Verification items for the finished model (mm, model axes). Face numbers are marked on the shaded views. A direction names the side the tool comes from. Give positions to 0.01 mm unless a question says otherwise; leave off trailing zeros. Order: outer loops, then holes, each group sorted by start corner. A loop starts at its lowest first (then second) coordinate and runs counter-clockwise, first axis right, second up. Notation, with made-up numbers: (25.5, 15.5) -> (66.5, 15.5) arc R19 ccw to (66.5, 41.5) -> close; hole circle Ø4 at (33, -15). An arc over 180 degrees is marked (long way). Return JSON: item names as keys, results as strings. Group by question number.
(1) Cross-section at D-D on z = 52. Enter the section's corners in (x, y).
(2) Cross-section at B-B on x = -13.5. Enter the section's corners in (y, z), then the cut area to 3 significant figures.
(3) Thickness scan on line 1 along Z through (x, y) = (-22.75, 37); line 2 along Y through (x, z) = (-16.75, 18); line 3 along Y through (x, z) = (-19.75, 10). Record the ranges inside material, lowest first.
(4) Cross-section at A-A on y = 11. Enter the section's corners in (x, z), then the cut area to 3 significant figures.
(5) Depth check by flat-ended pin: pin 1 Ø2 at (x, z) = (-17.5, 43.5) entering from +Y; pin 2 Ø9 at (x, y) = (-16.19, 27.83) entering from -Z; pin 3 Ø5 at (x, z) = (-17, 16.5) entering from +Y; pin 4 Ø12 at (x, z) = (-25, 61.5) entering from +Y. Enter the tip coordinate at first touch or a pass-through.
(6) Cross-section at C-C on z = 5. Enter the section's corners in (x, y), then the cut area to 3 significant figures.
(7) Tool access check on the marked faces 1 and 2. Record the directions out of +Z, -Z, +X, -X, +Y, -Y that give a thin tool (end or side, any length) a straight path to the whole face; none if there is none.
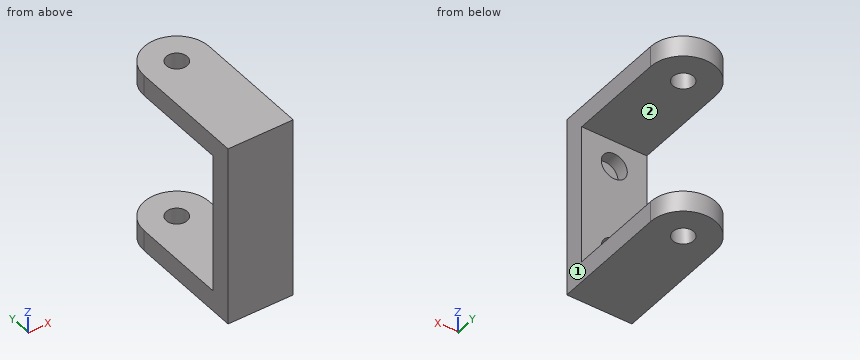
from build123d import *

# Parameters (mm, degrees)
IZIM1_W                     = 25
IZIM1_H                     = 57.5
Y_KSEKLIK_EKSTR_ZYON1_DEPTH = 70
RADYUS1_RADIUS              = 12.5
RADYUS1_LENGTH              = 70
IZIM3_W                     = 54
IZIM3_H                     = 49.5
KES_EKSTR_ZYON1_DEPTH       = 85.564510613
IZIM4_R                     = 5
KES_EKSTR_ZYON2_DEPTH       = 5
IZIM5_R                     = 4
KES_EKSTR_ZYON3_DEPTH       = 86.728971246


with BuildPart() as part:
    # Çizim1 → Yükseklik-Ekstrüzyon1 (new body)
    with BuildSketch(Plane.XY):
        with Locations((-16.193205739, 11.575630252)):
            Rectangle(IZIM1_W, IZIM1_H)
    extrude(amount=Y_KSEKLIK_EKSTR_ZYON1_DEPTH)

    # Radyus1: full round fillet: the end face becomes a half cylinder, R = half its width
    radyus1_face = Plane((-16.193205739, 40.325630252, 35), x_dir=(0, 0, 1), z_dir=(0, 1, 0))  # on the end face: x along it, z out of the body
    radyus1_slab = radyus1_face.offset(-RADYUS1_RADIUS / 2) * Box(RADYUS1_LENGTH, 2 * RADYUS1_RADIUS, RADYUS1_RADIUS, mode=Mode.PRIVATE)  # the body's end, R deep
    radyus1_round = Plane((-16.193205739, 27.825630252, 35), x_dir=(0, 1, 0), z_dir=(0, 0, 1)) * Cylinder(RADYUS1_RADIUS, RADYUS1_LENGTH, mode=Mode.PRIVATE)  # its axis R under the face
    add(radyus1_slab - radyus1_round, mode=Mode.SUBTRACT)

    # Çizim3 → Kes-Ekstrüzyon1 (cut, through all)
    with BuildSketch(Plane(origin=(-3.693205739, 0, 0), x_dir=(0, 0, -1), z_dir=(1, 0, 0))):
        with Locations((-35, 15.575630252)):
            Rectangle(IZIM3_W, IZIM3_H)
    extrude(amount=-KES_EKSTR_ZYON1_DEPTH, mode=Mode.SUBTRACT)

    # Çizim4 → Kes-Ekstrüzyon2 (cut)
    with BuildSketch(Plane(origin=(0, -9.174369748, 0), x_dir=(1, 0, 0), z_dir=(0, 1, 0))):
        with Locations(Location((-16.193205739, -18, 0), (0, 0, 180))):
            Circle(IZIM4_R)
        with Locations(Location((-16.193205739, -52, 0), (0, 0, 180))):
            Circle(IZIM4_R)
    extrude(amount=-KES_EKSTR_ZYON2_DEPTH, mode=Mode.SUBTRACT)

    # Çizim5 → Kes-Ekstrüzyon3 (cut, through all)
    with BuildSketch(Plane.XY.offset(70)):
        with Locations((-16.193205739, 27.825630252)):
            Circle(IZIM5_R)
    extrude(amount=-KES_EKSTR_ZYON3_DEPTH, mode=Mode.SUBTRACT)


solid = part.part
Verdict:
{
 "1": {"outline": "(-28.69, -17.17) -> (-3.69, -17.17) -> (-3.69, -9.17) -> (-11.19, -9.17) -> (-11.19, -14.17) -> (-21.19, -14.17) -> (-21.19, -9.17) -> (-28.69, -9.17) -> close"},
 "2": {"outline": "(-17.17, 0) -> (24.87, 0) -> (24.87, 8) -> (-9.17, 8) -> (-9.17, 13.79) -> (-14.17, 13.79) -> (-14.17, 22.21) -> (-9.17, 22.21) -> (-9.17, 47.79) -> (-14.17, 47.79) -> (-14.17, 56.21) -> (-9.17, 56.21) -> (-9.17, 62) -> (24.87, 62) -> (24.87, 70) -> (-17.17, 70) -> close; (30.78, 0) -> (40.03, 0) -> (40.03, 8) -> (30.78, 8) -> close; (30.78, 62) -> (40.03, 62) -> (40.03, 70) -> (30.78, 70) -> close", "area": "1,170 mm²"},
 "3": {"line 1": "0 to 8, 62 to 70", "line 2": "-17.17 to -14.17", "line 3": "-17.17 to -9.17"},
 "4": {"outline": "(-28.69, 0) -> (-3.69, 0) -> (-3.69, 8) -> (-28.69, 8) -> close; (-28.69, 62) -> (-3.69, 62) -> (-3.69, 70) -> (-28.69, 70) -> close", "area": "400 mm²"},
 "5": {"pin 1": "y = -9.17", "pin 2": "z = 0", "pin 3": "y = -14.17", "pin 4": "y = 40"},
 "6": {"outline": "(-28.69, -17.17) -> (-3.69, -17.17) -> (-3.69, 27.83) arc R12.5 ccw to (-28.69, 27.83) -> close; hole circle Ø8 at (-16.19, 27.83)", "area": "1,320 mm²"},
 "7": {"face 1": "+Z, -Z, +X, +Y, -Y", "face 2": "+X, -X, +Y"}
}
